from build123d import *

# Parameters (mm, degrees)
SKETCH1_R           = 15
BOSS_EXTRUDE1_DEPTH = 100
CHAMFER1_SIZE       = 2
SKETCH3_W           = 8
SKETCH3_H           = 60
CUT_EXTRUDE1_DEPTH  = 4
FILLET1_R           = 3


with BuildPart() as part:
    # Sketch1 → Boss-Extrude1 (new body)
    with BuildSketch(Plane.XY):
        Circle(SKETCH1_R)
    extrude(amount=BOSS_EXTRUDE1_DEPTH)

    # Chamfer1
    chamfer1_edges = [part.edges().sort_by_distance(p)[0] for p in [
        (-15, 0, 0),
    ]]
    chamfer(chamfer1_edges, length=CHAMFER1_SIZE)

    # Sketch3 → Cut-Extrude1 (cut)
    with BuildSketch(Plane(origin=(0, 15, 100), x_dir=(1, 0, 0), z_dir=(0, 1, 0))):
        with Locations((0, 70)):
            Rectangle(SKETCH3_W, SKETCH3_H)
    extrude(amount=-CUT_EXTRUDE1_DEPTH, mode=Mode.SUBTRACT)

    # Fillet1
    fillet1_edges = [part.edges().sort_by_distance(p)[0] for p in [
        (0, 11, 60),
    ]]
    fillet(fillet1_edges, radius=FILLET1_R)


solid = part.part
The model under review builds one solid part; all positions refer to its coordinate system, in mm. A direction names the side the tool comes from. Give positions to 0.01 mm unless a question says otherwise; leave off trailing zeros. Order: outer loops, then holes, each group sorted by start corner. A loop starts at its lowest first (then second) coordinate and runs counter-clockwise, first axis right, second up. Notation, with made-up numbers: M 26.5,34 L 75.5,34 A17 cw 75.5,67 Z; hole C 76,31.25 d9. An arc over 180 degrees is marked long. Answer in a Markdown table with one row per item. Add a question column.
1. For pin 1 Ø6 at (y, z) = (10.5, 20.5) entering from -X; pin 2 Ø1 at (y, z) = (12, 25.5) entering from +X; pin 3 Ø12 at (y, z) = (-7.5, 66) entering from -X, all flat-tipped, find the tip position at first contact; note any pin that passes through.
2. Mouldability with a two-part tool opening along X and no side actions: class faces 3 (the cylindrical face through (-3.252, -14.643, 50.314)), 4 (the flat face through (0, 0, 0)), 5 (the flat face through (4, 13, 30)) as released by +X, released by -X, zero draft, split by the parting line, or undercut.
3. Add section A-A on x = 0. State the section outline as (y, z) points, plus the area to 3 significant figures.
4. Add section B-B on z = 23. State the section outline as (x, y) points, plus the area to 3 significant figures.
5. To check wall thickness, follow line 1 along Y through (x, z) = (7.5, 39.5); line 2 along X through (y, z) = (-0.75, 44.5); line 3 along X through (y, z) = (-5.25, 19). State the ranges of each line that lie inside material, in increasing order.
6. Machinability: for faces 1 (the cylindrical face through (0.06, 11.86, 59.1)), 2 (the flat face through (0, 0, 100)), which of the approach directions +Z, -Z, +X, -X, +Y, -Y give a long, thin tool a straight path to every point of the face, cutting with its end or side? Answer none if there is none.
7. Add section C-C on z = 72. State the section outline as (x, y) points.
The answers:
| question | item | result |
|---|---|---|
| 1 | pin 1 | x = -12.99 |
| 1 | pin 2 | x = 9.63 |
| 1 | pin 3 | x = -14.92 |
| 2 | face 3 | split by the parting line |
| 2 | face 4 | zero draft |
| 2 | face 5 | undercut |
| 3 | outline | M -15,2 L -13,0 L 11,0 L 11,57 A3 cw 14,60 L 15,60 L 15,100 L -15,100 Z |
| 3 | area | 2,760 mm2 |
| 4 | outline | M -4,11 L -4,14.46 A15 ccw long 4,14.46 L 4,11 Z |
| 4 | area | 676 mm2 |
| 5 | line 1 | -12.99 to 12.99 |
| 5 | line 2 | -14.98 to 14.98 |
| 5 | line 3 | -14.05 to 14.05 |
| 6 | face 1 | -Z, +Y |
| 6 | face 2 | +Z, +X, -X, +Y, -Y |
| 7 | outline | C 0,0 d30 |
